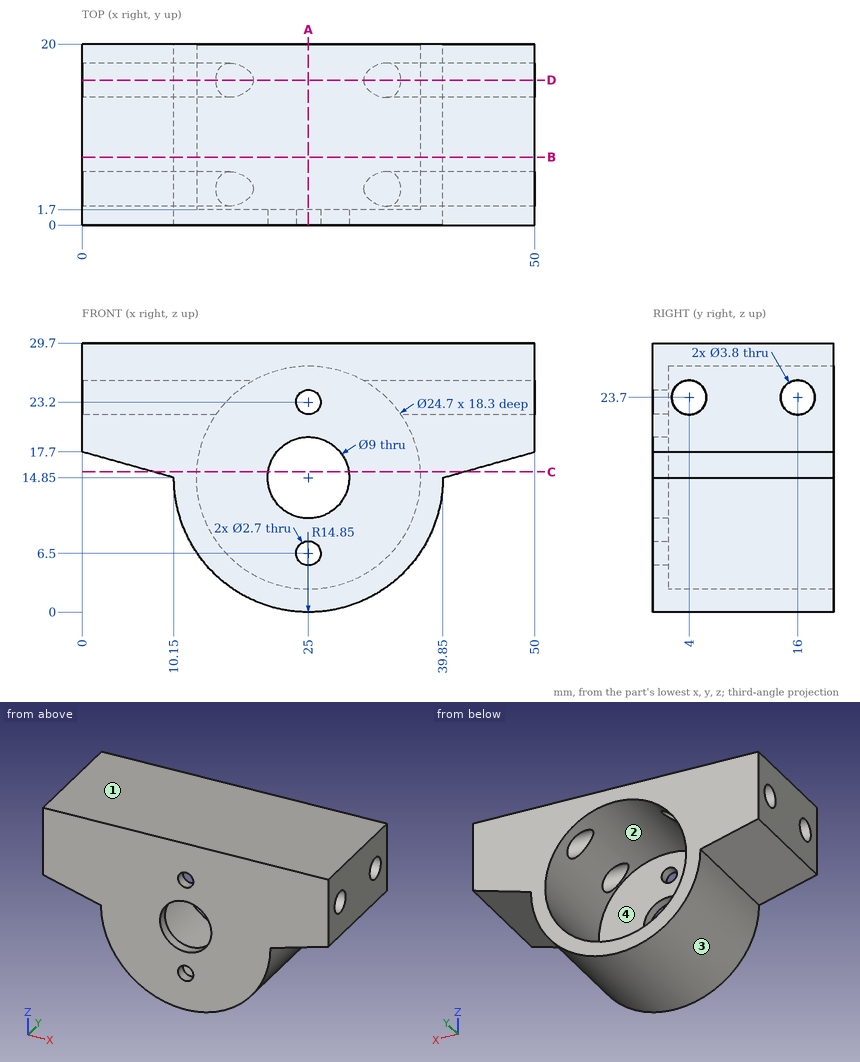
For this review, use the dimensioned drawing (mm, ordinates from the lowest corner) and the shaded views. Give positions to 0.01 mm unless a question says otherwise; leave off trailing zeros. Loops run counter-clockwise (first coordinate to the right, second up) from the corner with the lowest first, then second, coordinate; pieces in that order, holes last.
Item 1: Insertion check: pin 1 (1.5 mm diameter, centred on y = 17, z = 5, fed in from +X); pin 2 (3 mm diameter, centred on x = 25, z = 6.5, fed in from +Y). Each pin has a flat end and moves straight along its axis. Give the tip position at first contact, or say it passes through.
Item 2: Take a section at C-C, the plane z = 15.5. State the section outline as (x, y) points.
Item 3: Take a section at D-D, the plane y = 16. State the section outline as (x, z) points, and give its area (3 significant figures).
Item 4: For line 1 along Y through (x, z) = (6, 23.7); line 2 along X through (y, z) = (0.85, 23.2); line 3 along Y through (x, z) = (42, 23), list the stretches that pass through material, from the lowest coordinate up.
Item 5: Take a section at A-A, the plane x = 25. State the section outline as (y, z) points.
Item 6: Take a section at B-B, the plane y = 7.5. State the section outline as (x, z) points, and give its area (3 significant figures).
Item 7: Draft analysis for pull direction X (two halves, no side actions). For the marked faces 1, 2, 3 and 4, state which applies: +X half, -X half, draft (parallel to the pull), parting line (faces both ways), or undercut.
Calculated:
1. pin 1: stops at x = 36.74
1. pin 2: stops at y = 1.7
2. outline: (7.84, 0) - (20.55, 0) - (20.55, 1.7) - (12.67, 1.7) - (12.67, 20) - (7.84, 20) - close; (29.45, 0) - (42.16, 0) - (42.16, 20) - (37.33, 20) - (37.33, 1.7) - (29.45, 1.7) - close
3. outline: (0, 17.7) - (10.15, 14.85) arc R14.85 ccw to (39.85, 14.85) - (50, 17.7) - (50, 21.8) - (35.21, 21.8) arc R12.35 cw (long way) to (14.79, 21.8) - (0, 21.8) - close; (0, 25.6) - (18.92, 25.6) arc R12.35 cw to (31.08, 25.6) - (50, 25.6) - (50, 29.7) - (0, 29.7) - close
3. area: 455 mm2
4. line 1: y = 0 to 2.1, 5.9 to 14.1, 17.9 to 20
4. line 2: x = 0 to 23.65, 26.35 to 50
4. line 3: y = 0 to 2.23, 5.77 to 14.23, 17.77 to 20
5. outline: (0, 0) - (20, 0) - (20, 2.5) - (1.7, 2.5) - (1.7, 5.15) - (0, 5.15) - close; (0, 7.85) - (1.7, 7.85) - (1.7, 10.35) - (0, 10.35) - close; (0, 19.35) - (1.7, 19.35) - (1.7, 21.85) - (0, 21.85) - close; (0, 24.55) - (1.7, 24.55) - (1.7, 27.2) - (20, 27.2) - (20, 29.7) - (0, 29.7) - close
6. outline: (0, 17.7) - (10.15, 14.85) arc R14.85 ccw to (39.85, 14.85) - (50, 17.7) - (50, 29.7) - (0, 29.7) - close; hole circle Ø24.7 at (25, 14.85)
6. area: 581 mm2
7. face 1: draft
7. face 2: undercut
7. face 3: parting line
7. face 4: undercut
